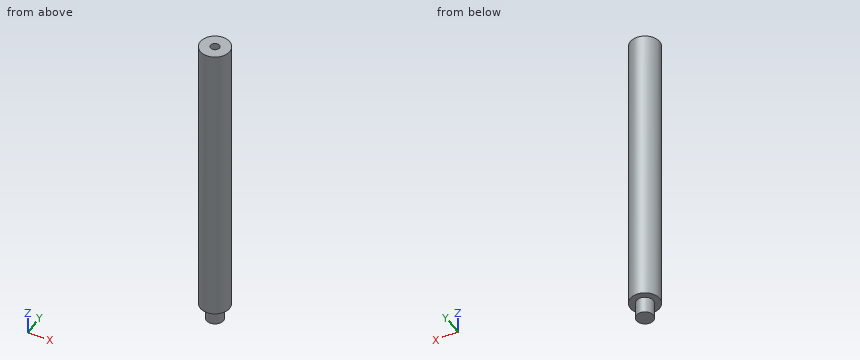
Autodesk Inventor part; units mm, degrees
ref_plane "YZ Plane" through (0, 0, 0) normal (1, 0, 0) x (0, 1, 0)
ref_plane "XZ Plane" through (0, 0, 0) normal (0, 1, 0) x (-1, 0, 0)
ref_plane "XY Plane" through (0, 0, 0) normal (0, 0, 1) x (1, 0, 0)
sketch "Sketch1" plane through (0, 0, 0) normal (0, 0, 1) x (1, 0, 0)
  circle A0 centre (0, 0) radius 19.05
  dimension "d0" = 38.1
extrude "Extrusion1" add sketch "Sketch1" along normal blind 381
sketch "Sketch2" plane through (0, 0, 381) normal (0, 0, 1) x (1, 0, 0)
  circle A0 centre (0, 0) radius 5.715
  dimension "d3" = 11.43
extrude "Extrusion2" cut sketch "Sketch2" against normal blind 317.5
sketch "Sketch3" plane through (0, 0, 0) normal (0, 0, -1) x (-1, 0, 0)
  circle A0 centre (0, 0) radius 10.9855
  dimension "d6" = 21.971
extrude "Extrusion3" add sketch "Sketch3" along normal blind 21.59
thread "Thread1"
properties part number "Cylinder 1"
Part model, mm, in its own coordinate system. Coordinates: 2 decimals unless noted, no trailing zeros. Order: outer loops, then holes, each group sorted by start corner. A loop starts at its lowest first (then second) coordinate and runs counter-clockwise, first axis right, second up. Notation, with made-up numbers: M 66,0 L 98,0 A30 cw 98,31 Z; hole C 70,84 d6. An arc over 180 degrees is marked long. One line per question, with ' | ' between items.
Q1. Slice it at C-C (z = 90.5). Give the cut face in (x, y) (3 decimals), and give its area (3 significant figures).
A:
outline: C 0,0 d38.1; hole C 0,0 d11.43 | area: 1,040 mm^2
Q2. Drill centre lines: line 1 (Y direction, x = 0, z = 209) (3 decimals); line 2 (Z direction, x = 16.5, y = -8.5); line 3 (X direction, y = -4, z = 333). Where is each one in solid material? Low to high.
A:
line 1: y = -19.05 to -5.715, 5.715 to 19.05 | line 2: z = 0 to 381 | line 3: x = -18.63 to -4.08, 4.08 to 18.63
Q3. Pin check, flat tips, straight feed: P1, Ø2, axis at x = 6.5, z = 84, coming from the -Y side; P2, Ø3.5, axis at x = 2.5, y = -0.5, coming from the +Z side; P3, Ø6, axis at x = 2.5, z = 115, coming from the -Y side. Stop position of each tip, or through.
A:
P1: stops at y = -18.24 | P2: stops at z = 63.5 | P3: stops at y = -19.05
